Here's how the part is built. I have some questions about the finished solid (model axes, mm). Give positions to 0.01 mm unless a question says otherwise; leave off trailing zeros. Order: outer loops, then holes, each group sorted by start corner. A loop starts at its lowest first (then second) coordinate and runs counter-clockwise, first axis right, second up.
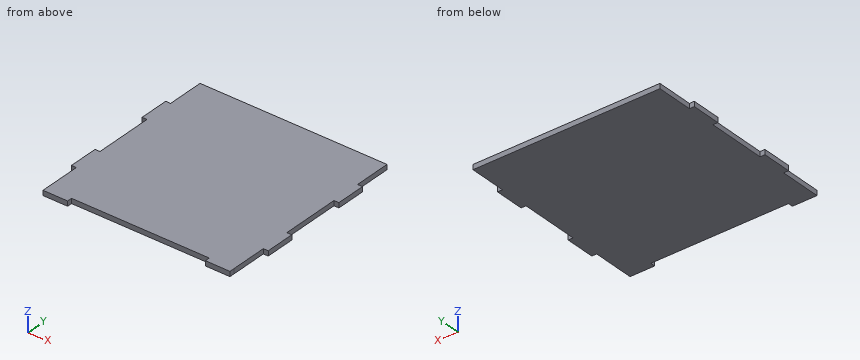
from build123d import *

# Parameters (mm, degrees)
F0_W      = 101.6
F0_H      = 101.6
F1_DEPTH  = 2.54
F3_DEPTH  = 2.54
F4_W      = 2.54
F4_H      = 16.51
F4_H_2    = 30.48
F4_H_3    = 21.59
F5_DEPTH  = 25.4
F6_W      = 8.149925
F6_H      = 6.423097
F6_W_2    = 6.710898
F7_DEPTH  = 25.4
F8_W      = 12.7
F8_H      = 2.54
F9_DEPTH  = 2.54
F10_W     = 2.54
F10_H     = 2.54
F11_DEPTH = 2.54
F12_W     = 2.54
F12_H     = 2.54
F13_DEPTH = 25.4


with BuildPart() as f1:
    # F0 (on Top) → F1 (new body)
    with BuildSketch(Plane.XY):
        Rectangle(F0_W, F0_H)
    extrude(amount=F1_DEPTH)

    # F2 (on face) → F3 (cut)
    with BuildSketch(Plane.XZ.offset(50.8)):
        Polygon((-41.91, 2.54), (-39.37, 0), (39.37, 0), (41.91, 2.54), align=None)
    extrude(amount=-F3_DEPTH, mode=Mode.SUBTRACT)

    # F4 (on face) → F5 (cut)
    with BuildSketch(Plane.XY.offset(2.54)):
        with Locations((-49.53, -40.005)):
            Rectangle(F4_W, F4_H)
        with Locations((-49.53, -1.27)):
            Rectangle(F4_W, F4_H_2)
        with Locations((-49.53, 40.005)):
            Rectangle(F4_W, F4_H_3)
        with Locations((49.53, -40.005)):
            Rectangle(F4_W, F4_H)
        with Locations((49.53, -1.27)):
            Rectangle(F4_W, F4_H_2)
        with Locations((49.53, 40.005)):
            Rectangle(F4_W, F4_H_3)
    extrude(amount=-F5_DEPTH, mode=Mode.SUBTRACT)

    # F6 (on face) → F7 (cut)
    with BuildSketch(Plane.XY.offset(2.54)):
        with Locations((52.334962, -51.471548)):
            Rectangle(F6_W, F6_H)
        with Locations((-51.615449, -51.471548)):
            Rectangle(F6_W_2, F6_H)
    extrude(amount=-F7_DEPTH, mode=Mode.SUBTRACT)

    # F8 (on face) → F9 (join)
    with BuildSketch(Plane.XY.offset(2.54)):
        with Locations((41.91, -49.53)):
            Rectangle(F8_W, F8_H)
        with Locations((-41.91, -49.53)):
            Rectangle(F8_W, F8_H)
    extrude(amount=-F9_DEPTH)

    # F10 (on face) → F11 (join)
    with BuildSketch(Plane.XY.offset(2.54)):
        with Locations((-49.53, 30.48)):
            Rectangle(F10_W, F10_H)
        with Locations((-49.53, -15.24)):
            Rectangle(F10_W, F10_H)
        with Locations((49.53, -15.24)):
            Rectangle(F10_W, F10_H)
        with Locations((49.53, 30.48)):
            Rectangle(F10_W, F10_H)
    extrude(amount=-F11_DEPTH)

    # F12 (on face) → F13 (cut)
    with BuildSketch(Plane.XY.offset(2.54)):
        with Locations((49.53, -30.48)):
            Rectangle(F12_W, F12_H)
        with Locations((49.53, 15.24)):
            Rectangle(F12_W, F12_H)
        with Locations((-49.53, -30.48)):
            Rectangle(F12_W, F12_H)
        with Locations((-49.53, 15.24)):
            Rectangle(F12_W, F12_H)
    extrude(amount=-F13_DEPTH, mode=Mode.SUBTRACT)


solid = f1.part
Q1. If we section it at C-C on y = -39.5: List the corners of the cut face in (x, z) for me, plus the area to 3 significant figures.
Filled sheet:
outline: (-48.26, 0) - (48.26, 0) - (48.26, 2.54) - (-48.26, 2.54) - close
area: 245 mm2
Q2. I need wall thicknesses on L1, parallel to Y at x = -26, z = 0.45; L2, parallel to X at y = -38, z = 0.75. Which ranges of each line are inside material? Lowest first, please.
Filled sheet:
L1: y = -48.26 to 50.8
L2: x = -48.26 to 48.26
Q3. If we section it at B-B on x = 9.5: List the corners of the cut face in (y, z) for me.
Filled sheet:
outline: (-48.26, 0) - (50.8, 0) - (50.8, 2.54) - (-48.26, 2.54) - close
Q4. I'm going to push flat-ended pins straight in: P1, Ø0.8, axis at x = -49.5, z = 1, coming from the -Y side; P2, Ø1.3, axis at y = -49.5, z = 1, coming from the +X side; P3, Ø0.8, axis at x = -49, z = 2, coming from the +Y side. Where does each tip first touch, or does it pass through?
Filled sheet:
P1: stops at y = -29.21
P2: stops at x = 48.26
P3: stops at y = 31.75
Q5. If we section it at A-A on z = 0.85: List the corners of the cut face in (x, y) for me, plus the area to 3 significant figures.
Filled sheet:
outline: (-50.8, -29.21) - (-48.26, -29.21) - (-48.26, -50.8) - (-35.56, -50.8) - (-35.56, -48.26) - (35.56, -48.26) - (35.56, -50.8) - (48.26, -50.8) - (48.26, -29.21) - (50.8, -29.21) - (50.8, -13.97) - (48.26, -13.97) - (48.26, 16.51) - (50.8, 16.51) - (50.8, 31.75) - (48.26, 31.75) - (48.26, 50.8) - (-48.26, 50.8) - (-48.26, 31.75) - (-50.8, 31.75) - (-50.8, 16.51) - (-48.26, 16.51) - (-48.26, -13.97) - (-50.8, -13.97) - close
area: 9,780 mm2
